The listing builds one solid part. Answer for the finished solid, in the listing's coordinates (mm). A direction names the side the tool comes from. Coordinates: 2 decimals unless noted, no trailing zeros. Loops run counter-clockwise (first coordinate to the right, second up) from the corner with the lowest first, then second, coordinate; pieces in that order, holes last. Notation, with made-up numbers: (-39.5, 48.5) - (12.5, 48.5) arc R8 ccw to (12.5, 59.5) - close; hole circle Ø6 at (12.5, 58.25). An arc over 180 degrees is marked (long way). Return JSON: item names as keys, results as strings. Group by question number.
1. The mould has two halves that part along X. Classify faces 1 (the face through (-55.47, 3.68, -10.21)), 2 (the face through (-27.6, 3.1, -5.1)), 3 (the face through (0, 3, -22)): pulls with the +X half, pulls with the -X half, needs draft (parallel to the pull), parting line crosses it, or undercut.
2. Section D-D (z = -21.59) is taken. Write down the section's boundary in (x, y).
3. Section B-B (x = -43) is taken. Write down the section's boundary in (y, z), and give its area (3 significant figures).
4. Section A-A (z = -6.09) is taken. Write down the section's boundary in (x, y), and give its area (3 significant figures).
5. Find the intervals of material crossed by line 1 along X through (y, z) = (3.25, -21.59); line 2 along Z through (x, y) = (-57.5, 5); line 3 along X through (y, z) = (3.25, -38.5), in increasing order.
6. Section C-C (y = 5.5) is taken. State how many separate pieces and enclosed holes the cut face has, and give its area (3 significant figures).
7. Which of the six approach directions +Z, -Z, +X, -X, +Y, -Y give full straight-line access (tool end or side, diameter ignored) to faces 4 (the face through (-55.49, 3.13, -36.26)), 5 (the face through (-55.47, 2.78, -30.49))?
Autodesk Inventor part; units mm, degrees
ref_plane "YZ Plane" through (0, 0, 0) normal (1, 0, 0) x (0, 1, 0)
ref_plane "XZ Plane" through (0, 0, 0) normal (0, 1, 0) x (-1, 0, 0)
ref_plane "XY Plane" through (0, 0, 0) normal (0, 0, 1) x (1, 0, 0)
sketch "Sketch1" plane through (0, 0, 0) normal (0, 1, 0) x (-1, 0, 0)
  line L0 (0, 0) -> (61.9125, 0)
  line L1 (61.9125, 0) -> (61.9125, -43.18)
  line L2 (61.9125, -43.18) -> (0, -43.18)
  line L3 (0, -43.18) -> (0, 0)
  dimension "d0" = 61.9125
  dimension "d1" = 43.18
extrude "Extrusion1" add sketch "Sketch1" along normal blind 6.35
sketch "Sketch2" plane through (0, 6.35, 0) normal (0, 1, 0) x (1, 0, 0)
  line L0 (-61.9125, 43.18) -> (-61.9125, 0)
  line L1 (-61.9125, 0) -> (0, 0)
  line L2 (0, 0) -> (0, 43.18)
  line L3 (-61.9125, 43.18) -> (0, 43.18)
  line L4 (-61.9125, 43.18) -> (-61.9125, 0)
  line L5 (0, 43.18) -> (-61.9125, 43.18)
  line L6 (-61.9125, 0) -> (0, 0)
  line L7 (0, 0) -> (0, 43.18)
  point P0 (-41.5925, 21.59)
  point P1 (-57.0925, 37.09)
  point P2 (-57.0925, 6.09)
  point P3 (-26.0925, 6.09)
  point P4 (-21.2725, 21.59)
  point P5 (-26.0925, 37.09)
  dimension "d4" = 6.09
  dimension "d5" = 4.82
  dimension "d6" = 6.09
  dimension "d7" = 4.82
  dimension "d8" = 6.09
  dimension "d9" = 26.0925
  dimension "d10" = 21.2725
  dimension "d11" = 21.59
  dimension "d12" = 6.09
  dimension "d13" = 26.0925
  dimension "d14" = 21.59
  dimension "d15" = 20.32
hole "Hole1" at (-57.0925, 6.35, -37.09) at (-57.0925, 6.35, -6.09) at (-26.0925, 6.35, -6.09) at (-26.0925, 6.35, -37.09) direction (0, -1, 0) diameter 3.6068 depth 10.9728 tip angle 118
hole "Hole2" at (-41.5925, 6.35, -21.59) direction (0, -1, 0) diameter 10.1001 depth 10.9728 tip angle 118
sketch "Sketch3" plane through (-61.9125, 0, -43.18) normal (-1, 0, 0) x (0, 0, 1)
  line L0 (0, 0) -> (0, 6.35)
  line L1 (43.18, 0) -> (43.18, 6.35)
  line L2 (0, 6.35) -> (43.18, 6.35)
  point P0 (11.43, 3.175)
  point P1 (31.75, 3.175)
  dimension "d37" = 11.43
  dimension "d38" = 11.43
  dimension "d39" = 3.175
hole "Hole3" at (-61.9125, 3.175, -31.75) at (-61.9125, 3.175, -11.43) direction (1, 0, 0) diameter 2.6416 depth 12.7 tip angle 118
hole "Hole4" at (-21.2725, 6.35, -21.59) direction (0, -1, 0) diameter 6.35 depth 10.9728 tip angle 118
properties part number "AR-BracketLeft2"
The answers:
{
 "1": {"face 1": "needs draft", "face 2": "undercut", "face 3": "pulls with the +X half"},
 "2": {"outline": "(-61.91, 0) - (-46.64, 0) - (-46.64, 6.35) - (-61.91, 6.35) - close; (-36.54, 0) - (-24.45, 0) - (-24.45, 6.35) - (-36.54, 6.35) - close; (-18.1, 0) - (0, 0) - (0, 6.35) - (-18.1, 6.35) - close"},
 "3": {"outline": "(0, -43.18) - (6.35, -43.18) - (6.35, -26.44) - (0, -26.44) - close; (0, -16.74) - (6.35, -16.74) - (6.35, 0) - (0, 0) - close", "area": "213 mm2"},
 "4": {"outline": "(-61.91, 0) - (-58.9, 0) - (-58.9, 6.35) - (-61.91, 6.35) - close; (-55.29, 0) - (-27.9, 0) - (-27.9, 6.35) - (-55.29, 6.35) - close; (-24.29, 0) - (0, 0) - (0, 6.35) - (-24.29, 6.35) - close", "area": "347 mm2"},
 "5": {"line 1": "x = -61.91 to -46.64, -36.54 to -24.45, -18.1 to 0", "line 2": "z = -43.18 to -38.85, -35.33 to -7.85, -4.33 to 0", "line 3": "x = -61.91 to -58.22, -55.97 to -27.22, -24.97 to 0"},
 "6": {"separate pieces": "1", "enclosed holes": "6", "area": "2,520 mm2"},
 "7": {"face 4": "+Y, -Y", "face 5": "-X"}
}
